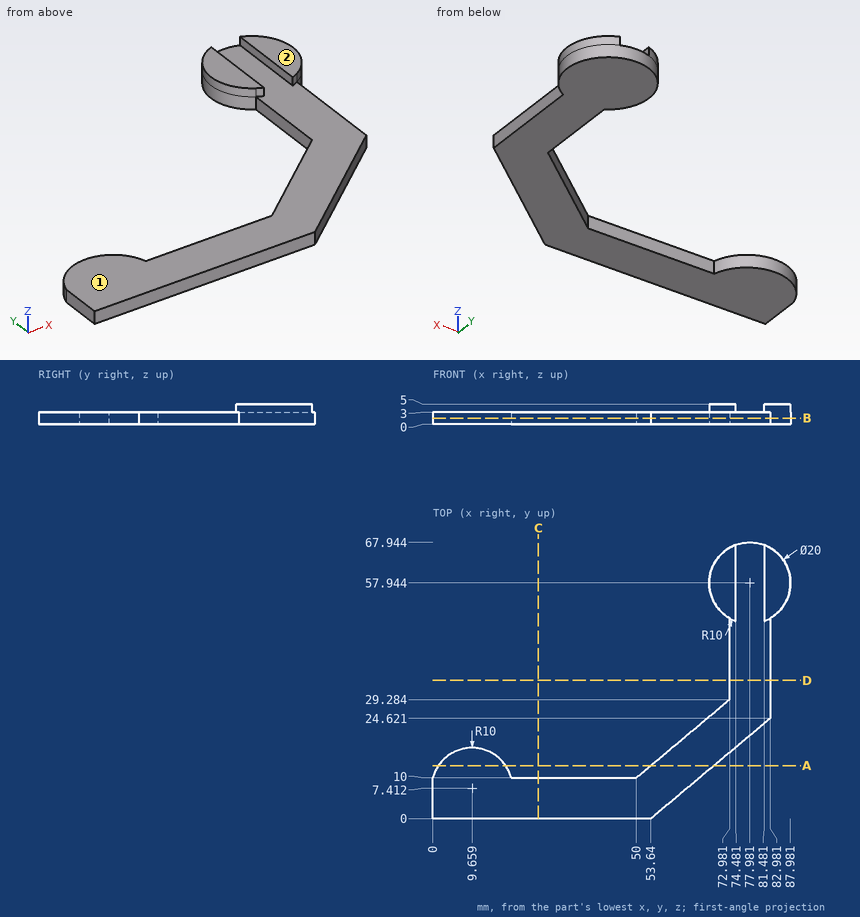
Geometry: see drawing. Coordinates: mm, zero at the bounding-box minimum. Coordinates: 2 decimals unless noted, no trailing zeros. Loops run counter-clockwise (first coordinate to the right, second up) from the corner with the lowest first, then second, coordinate; pieces in that order, holes last. Notation, with made-up numbers: M -13.5,23.5 L 9.5,23.5 A20 cw 9.5,36.5 Z; hole C 88,79.5 d6. An arc over 180 degrees is marked long. Answer in a Markdown table with one row per item.
Q1. Section B-B on z = 1.55. Return the cut outline in (x, y), plus the area to 3 significant figures.
Answers below:
| item | result |
|---|---|
| outline | M 0,0 L 53.64,0 L 82.98,24.62 L 82.98,49.28 A10 ccw long 72.98,49.28 L 72.98,29.28 L 50,10 L 19.32,10 A10 ccw 0,10 Z |
| area | 1,490 mm^2 |
Q2. Section D-D on y = 34. Return the cut outline in (x, z).
Answers below:
| item | result |
|---|---|
| outline | M 72.98,0 L 82.98,0 L 82.98,3 L 72.98,3 Z |
Q3. First-contact query: pin 1 (2.5 mm diameter, centred on y = 41, z = 1.5, fed in from -X); pin 2 (1.6 mm diameter, centred on y = 59, z = 4.5, fed in from +X); pin 3 (2.5 mm diameter, centred on y = 34, z = 1.5, fed in from +X). Flat tips, straight axial feed; report the tip coordinate or a pass-through.
Answers below:
| item | result |
|---|---|
| pin 1 | stops at x = 72.98 |
| pin 2 | stops at x = 87.98 |
| pin 3 | stops at x = 82.98 |
Q4. Ray query, probe 1 along Z at (x, y) = (67, 16); probe 2 along Y at (x, z) = (45, 1.45); probe 3 along X at (y, z) = (65.5, 3.45). Return the intervals inside material, ascending. Write a range as from..to.
Answers below:
| item | result |
|---|---|
| probe 1 | z = 0..3 |
| probe 2 | y = 0..10 |
| probe 3 | x = 71.43..74.48, 81.48..84.53 |
Q5. Section C-C on x = 26. Return the cut outline in (y, z).
Answers below:
| item | result |
|---|---|
| outline | M 0,0 L 10,0 L 10,3 L 0,3 Z |
Q6. Draft query along X for the marked faces 1 and 2. Return one class per face: pulls with the +X half, pulls with the -X half, needs draft (parallel to the pull), parting line crosses it, or undercut.
Answers below:
| item | result |
|---|---|
| face 1 | undercut |
| face 2 | needs draft |
Q7. Section A-A on y = 13. Return the cut outline in (x, z) (1 decimal).
Answers below:
| item | result |
|---|---|
| outline | M 1.4,0 L 18,0 L 18,3 L 1.4,3 Z; M 53.6,0 L 69.1,0 L 69.1,3 L 53.6,3 Z |
